```python
from build123d import *

# Parameters (mm, degrees)
F1_DEPTH = 9.525
F0_R     = 25.4
F2_DEPTH = 25.4
F0_R_2   = 17.4625
F3_DEPTH = 15.875


with BuildPart() as f1:
    # F0 (on Front) → F1 (new body, symmetric)
    with BuildSketch(Plane.XZ):
        with BuildLine():
            ThreePointArc((-23.4888751152, 42.803092487), (5.3509296025, 29.4999956791), (17.1177038322, 0))
            ThreePointArc((17.1177038322, 0), (5.3509296025, -29.4999956791), (-23.4888751152, -42.803092487))
            Line((-23.4888751152, -42.803092487), (156.9848090954, -33.2912941566))
            ThreePointArc((156.9848090954, -33.2912941566), (121.8927038322, 0), (156.9848090954, 33.2912941566))
            Line((156.9848090954, 33.2912941566), (-23.4888751152, 42.803092487))
        make_face()
    extrude(amount=F1_DEPTH, both=True)

    # F0 (on Front) → F2 (join, symmetric)
    with BuildSketch(Plane.XZ):
        with BuildLine():
            ThreePointArc((-23.4888751152, -42.803092487), (5.3509296025, -29.4999956791), (17.1177038322, 0))
            ThreePointArc((17.1177038322, 0), (5.3509296025, 29.4999956791), (-23.4888751152, 42.803092487))
            ThreePointArc((-23.4888751152, 42.803092487), (-68.6072961678, 0), (-23.4888751152, -42.803092487))
        make_face()
        with Locations((-25.7447961678, 0)):
            Circle(F0_R, mode=Mode.SUBTRACT)
    extrude(amount=F2_DEPTH, both=True)

    # F0 (on Front) → F3 (join, symmetric)
    with BuildSketch(Plane.XZ):
        with BuildLine():
            ThreePointArc((188.5677038322, 0), (179.4157683202, 22.9444410837), (156.9848090954, 33.2912941566))
            ThreePointArc((156.9848090954, 33.2912941566), (121.8927038322, 0), (156.9848090954, -33.2912941566))
            ThreePointArc((156.9848090954, -33.2912941566), (179.4157683202, -22.9444410837), (188.5677038322, 0))
        make_face()
        with Locations((155.2302038322, 0)):
            Circle(F0_R_2, mode=Mode.SUBTRACT)
    extrude(amount=F3_DEPTH, both=True)


solid = f1.part
```
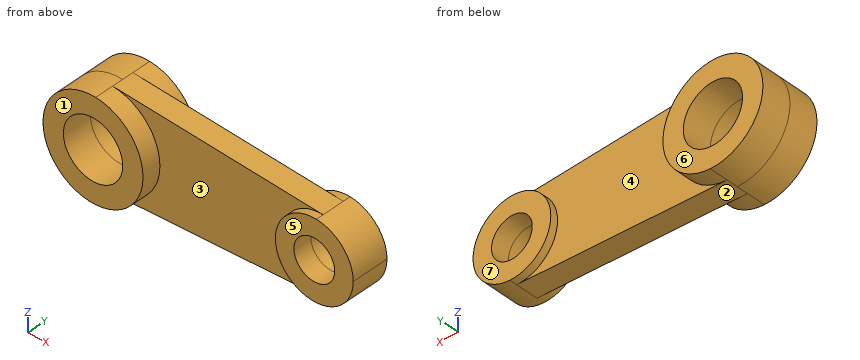
Source: CAD feature listing. Evaluate the final solid. Frame: model axes, mm. Face numbers are marked on the shaded views. A direction names the side the tool comes from. Give positions to 0.01 mm unless a question says otherwise; leave off trailing zeros. Write each loop counter-clockwise with the first axis right and the second up, starting at its lowest first coordinate (ties: lowest second). Pieces come first, ordered by that corner, then holes.
1. Section query C-C (y = -20). Return the cut outline in (x, z) (1 decimal), then the cut area to 3 significant figures.
2. Section query D-D (x = 58). Return the cut outline in (y, z) (3 decimals).
3. Section query B-B (z = -28.5). Return the cut outline in (x, y) (3 decimals).
4. Section query A-A (x = 166.5). Return the cut outline in (y, z) (3 decimals).
5. Pull-direction query (X, two-part tool) for the marked faces 1, 2, 3 and 4; classes: +X half, -X half, draft (parallel to the pull), parting line (faces both ways), or undercut.
6. Access query for the marked faces 5, 6 and 7. Directions: +Z, -Z, +X, -X, +Y, -Y. A direction counts if a zero-diameter tool reaches every point of the face in a straight line with its end or side. Return the directions, or none.
7. First-contact query: pin 1 (12 mm diameter, centred on y = 9.5, z = -25, fed in from -X); pin 2 (6 mm diameter, centred on y = 13.5, z = 12.5, fed in from +X); pin 3 (1 mm diameter, centred on x = 123, z = -15.5, fed in from -Y) (3 decimals). Flat tips, straight axial feed; report the tip coordinate or a pass-through.
8. Material intervals for line 1 along X through (y, z) = (14.5, -1); line 2 along X through (y, z) = (8, 7); line 3 along X through (y, z) = (-1, -5), sorted ascending.
Output values:
1. outline: circle Ø85.7 at (-25.7, 0); hole circle Ø50.8 at (-25.7, 0)
1. area: 3,740 mm2
2. outline: (-9.525, -38.508) - (9.525, -38.508) - (9.525, 38.508) - (-9.525, 38.508) - close
3. outline: (-57.76, -25.4) - (6.27, -25.4) - (6.27, -9.525) - (137.935, -9.525) - (137.935, -15.875) - (172.526, -15.875) - (172.526, 15.875) - (137.935, 15.875) - (137.935, 9.525) - (6.27, 9.525) - (6.27, 25.4) - (-57.76, 25.4) - close
4. outline: (-15.875, -31.375) - (15.875, -31.375) - (15.875, -13.339) - (-15.875, -13.339) - close; (-15.875, 13.339) - (15.875, 13.339) - (15.875, 31.375) - (-15.875, 31.375) - close
5. face 1: draft
5. face 2: +X half
5. face 3: undercut
5. face 4: undercut
6. face 5: +Z, -Z, +X, -Y
6. face 6: +Z, -Z, +X, -X, +Y
6. face 7: +Z, -Z, +X, +Y
7. pin 1: stops at x = -64.17
7. pin 2: stops at x = 187.19
7. pin 3: stops at y = -9.525
8. line 1: x = -68.6 to -51.13, -0.36 to 17.11, 121.91 to 137.8, 172.66 to 188.55
8. line 2: x = -68.03 to -50.16, -1.33 to 139.23, 171.23 to 187.82
8. line 3: x = -68.31 to -50.65, -0.84 to 138.5, 171.96 to 188.19
